```python
from build123d import *

# Parameters (mm, degrees)
F0_W     = 35
F0_H     = 20
F0_R     = 1.5
F1_DEPTH = 2.5
F2_W     = 35
F2_H     = 8
F2_H_2   = 2.5
F3_DEPTH = 3
F4_W     = 35
F4_H     = 2.5
F5_DEPTH = 10


with BuildPart() as f1:
    # F0 (on Front) → F1 (new body)
    with BuildSketch(Plane.XZ):
        with Locations((4.550226, 5.8339)):
            Rectangle(F0_W, F0_H)
        with Locations((-7.449774, 2.8339)):
            Circle(F0_R, mode=Mode.SUBTRACT)
        with Locations((16.550226, 2.8339)):
            Circle(F0_R, mode=Mode.SUBTRACT)
    extrude(amount=F1_DEPTH)

    # F2 (on face) → F3 (join)
    with BuildSketch(Plane.XY.offset(15.8339)):
        with Locations((4.550226, -6.5)):
            Rectangle(F2_W, F2_H)
        with Locations((4.550226, -1.25)):
            Rectangle(F2_W, F2_H_2)
    extrude(amount=F3_DEPTH)

    # F4 (on face) → F5 (join)
    with BuildSketch(Plane.XY.offset(18.8339)):
        with Locations((4.550226, -9.25)):
            Rectangle(F4_W, F4_H)
    extrude(amount=F5_DEPTH)


solid = f1.part
```
Input: part model. Units: mm. Frame: model coordinates. A direction names the side the tool comes from. Coordinates: 2 decimals unless noted, no trailing zeros. Order: outer loops, then holes, each group sorted by start corner. A loop starts at its lowest first (then second) coordinate and runs counter-clockwise, first axis right, second up. Notation, with made-up numbers: (33, -40) - (38, -40) arc R22 ccw to (38, -23) - close; hole circle Ø4 at (23.25, -9). An arc over 180 degrees is marked (long way). Put each result on its own line as item: value.
1. Cut plane A-A on x = 2. Return the cut outline in (y, z).
Report:
outline: (-10.5, 15.83) - (-2.5, 15.83) - (-2.5, -4.17) - (0, -4.17) - (0, 18.83) - (-8, 18.83) - (-8, 28.83) - (-10.5, 28.83) - close
2. Cut plane B-B on z = 11. Return the cut outline in (x, y).
Report:
outline: (-12.95, -2.5) - (22.05, -2.5) - (22.05, 0) - (-12.95, 0) - close
3. Contact query for flat-ended pins moving along their axis: pin 1 Ø3.5 at (x, z) = (16.55, 2.83) entering from -Y; pin 2 Ø4 at (x, y) = (-1.5, -4) entering from +Z; pin 3 Ø4 at (x, y) = (4.5, -7) entering from -Z. Output: stop coordinate, or through.
Report:
pin 1: stops at y = -2.5
pin 2: stops at z = 18.83
pin 3: stops at z = 15.83
4. Cut plane D-D on y = -1.25. Return the cut outline in (x, z), then the cut area to 3 significant figures.
Report:
outline: (-12.95, -4.17) - (22.05, -4.17) - (22.05, 18.83) - (-12.95, 18.83) - close; hole circle Ø3 at (-7.45, 2.83); hole circle Ø3 at (16.55, 2.83)
area: 791 mm2
5. Line query: line 1 along Y through (x, z) = (12, 8.5); line 2 along Y through (x, z) = (-11, 24); line 3 along Z through (x, y) = (20, -7.25). Output: solid intervals per line, ascending.
Report:
line 1: y = -2.5 to 0
line 2: y = -10.5 to -8
line 3: z = 15.83 to 18.83
6. Cut plane C-C on y = -4.75. Return the cut outline in (x, z), then the cut area to 3 significant figures.
Report:
outline: (-12.95, 15.83) - (22.05, 15.83) - (22.05, 18.83) - (-12.95, 18.83) - close
area: 105 mm2
7. Reachability of faces 1 (the face through (4, -10.5, 22)), 2 (the face through (4, -6, 15.834)), 3 (the face through (4, -8, 24)) from +Z, -Z, +X, -X, +Y, -Y: full face, straight path, thin tool, end or side. Return the list, or none.
Report:
face 1: +Z, -Z, +X, -X, -Y
face 2: -Z, +X, -X, -Y
face 3: +Z, +X, -X, +Y
8. Draft query along X for faces 4 (the face through (4, -9, 28.834)), 5 (the face through (17.936, -1.232, 2.259)), 6 (the face through (22.05, -4, 16)), 7 (the face through (-8.64, -1.23, 1.92)). Return one class per face: pulls with the +X half, pulls with the -X half, needs draft (parallel to the pull), parting line crosses it, or undercut.
Report:
face 4: needs draft
face 5: undercut
face 6: pulls with the +X half
face 7: undercut
